from build123d import *

# Parameters (mm, degrees)
SKETCH1_R           = 275
BOSS_EXTRUDE1_DEPTH = 70
SKETCH2_R           = 275
SKETCH2_R_2         = 265
CUT_EXTRUDE1_DEPTH  = 10
SKETCH3_R           = 275
BOSS_EXTRUDE2_DEPTH = 50
SKETCH4_R           = 150
SKETCH4_R_2         = 100
BOSS_EXTRUDE3_DEPTH = 100
BOSS_EXTRUDE4_DEPTH = 100
FILLET3_R           = 20
BOSS_EXTRUDE5_DEPTH = 75
CUT_EXTRUDE4_DEPTH  = 150
CUT_EXTRUDE5_DEPTH  = 87.5


with BuildPart() as part:
    # Sketch1 → Boss-Extrude1 (new body)
    with BuildSketch(Plane.XY):
        Circle(SKETCH1_R)
    extrude(amount=BOSS_EXTRUDE1_DEPTH)

    # Sketch2 → Cut-Extrude1 (cut)
    with BuildSketch(Plane.XY.offset(70)):
        Circle(SKETCH2_R)
        Circle(SKETCH2_R_2, mode=Mode.SUBTRACT)
    extrude(amount=-CUT_EXTRUDE1_DEPTH, mode=Mode.SUBTRACT)

    # Sketch3 → Boss-Extrude2 (add)
    with BuildSketch(Plane.XY.offset(70)):
        Circle(SKETCH3_R)
    extrude(amount=BOSS_EXTRUDE2_DEPTH)



with BuildPart() as body_2:
    # Sketch4 → Boss-Extrude3 (new body, symmetric)
    with BuildSketch(Plane(origin=(0, 0, 0), x_dir=(0, 0, -1), z_dir=(1, 0, 0))):
        with Locations((-375, 0)):
            Circle(SKETCH4_R)
        with Locations((-375, 0)):
            Circle(SKETCH4_R_2, mode=Mode.SUBTRACT)
    extrude(amount=BOSS_EXTRUDE3_DEPTH, both=True)


with BuildPart() as part_1:
    add(part.part)

    add(body_2.part)  # Boss-Extrude4 merges body 2
    # Sketch6 → Boss-Extrude4 (add, symmetric)
    with BuildSketch(Plane(origin=(0, 0, 0), x_dir=(0, 0, -1), z_dir=(1, 0, 0))):
        with BuildLine():
            Line((-375, 150), (-120, 150))
            Line((-120, 150), (-120, -150))
            Line((-120, -150), (-375, -150))
            ThreePointArc((-375, -150), (-225, 0), (-375, 150))
        make_face()
    extrude(amount=BOSS_EXTRUDE4_DEPTH, both=True)

    # Fillet3
    fillet3_edges = [part_1.edges().sort_by_distance(p)[0] for p in [
        (-100, -150, 247.5),
        (-100, 150, 247.5),
        (100, -150, 247.5),
        (100, 150, 247.5),
        (-100, 0, 525),
        (100, 0, 525),
    ]]
    fillet(fillet3_edges, radius=FILLET3_R)

    # Sketch7 → Boss-Extrude5 (add)
    with BuildSketch(Plane.XY.offset(120)):
        with BuildLine():
            ThreePointArc((-266.057108103, 69.560155462), (-275, 0), (-266.057108103, -69.560155462))
            Line((-266.057108103, -69.560155462), (-100, -130))
            Line((-100, -130), (-100, 130))
            Line((-100, 130), (-266.057108103, 69.560155462))
        make_face()
        with BuildLine():
            Line((100, -130), (266.057108103, -69.560155462))
            ThreePointArc((266.057108103, -69.560155462), (272.755114277, -35.066331942), (275, 0))
            ThreePointArc((275, 0), (272.755114277, 35.066331942), (266.057108103, 69.560155462))
            Line((266.057108103, 69.560155462), (100, 130))
            Line((100, 130), (100, -130))
        make_face()
        with BuildLine():
            ThreePointArc((35.333334581, 272.72065464), (0, 275), (-35.333334581, 272.72065464))
            Line((-35.333334581, 272.72065464), (-80, 150))
            Line((-80, 150), (80, 150))
            Line((80, 150), (35.333334581, 272.72065464))
        make_face()
        with BuildLine():
            Line((80, -150), (-80, -150))
            Line((-80, -150), (-35.333334581, -272.72065464))
            ThreePointArc((-35.333334581, -272.72065464), (0, -275), (35.333334581, -272.72065464))
            Line((35.333334581, -272.72065464), (80, -150))
        make_face()
    extrude(amount=BOSS_EXTRUDE5_DEPTH)

    # Sketch8 → Cut-Extrude4 (cut, symmetric)
    with BuildSketch(Plane(origin=(0, 0, 0), x_dir=(1, 0, 0), z_dir=(0, 1, 0))):
        Polygon((-300, -120), (-100, -195), (-300, -195), align=None)
        Polygon((300, -120), (100, -195), (300, -195), align=None)
    extrude(amount=CUT_EXTRUDE4_DEPTH, both=True, mode=Mode.SUBTRACT)

    # Sketch9 → Cut-Extrude5 (cut, symmetric)
    with BuildSketch(Plane(origin=(0, 0, 0), x_dir=(0, 0, -1), z_dir=(1, 0, 0))):
        Polygon((-195, 150), (-195, 290), (-120, 290), align=None)
        Polygon((-120, -290), (-195, -150), (-195, -290), align=None)
    extrude(amount=CUT_EXTRUDE5_DEPTH, both=True, mode=Mode.SUBTRACT)


solid = part_1.part
Verification items for the finished model (mm, model axes). A direction names the side the tool comes from. Give positions to 0.01 mm unless a question says otherwise; leave off trailing zeros. Write each loop counter-clockwise with the first axis right and the second up, starting at its lowest first coordinate (ties: lowest second). Pieces come first, ordered by that corner, then holes. Notation, with made-up numbers: (-8, 22.25) - (14, 22.25) arc R32 cw to (14, 56.25) - close; hole circle Ø2 at (83.25, 23.25). An arc over 180 degrees is marked (long way). Answer as CSV lines item,"result". Start each with the question number.
1. Sectioned sample at C-C (y = 161.5). Record the boundary of the cut face in (x, z), then the cut area to 3 significant figures.
2. Sectioned sample at A-A (x = 0). Record the boundary of the cut face in (y, z), then the cut area to 3 significant figures.
3. Depth check by flat-ended pin: pin 1 (1 mm diameter, centred on y = 189.5, z = 64, fed in from +X); pin 2 (1 mm diameter, centred on x = 26.5, z = 380.5, fed in from -Y); pin 3 (1 mm diameter, centred on x = -28.5, y = -108, fed in from +Z). Enter the tip coordinate at first touch or a pass-through.
4. Draft check along Z on faces 5 (the face through (-1.4, -60.848, 454.357)), 6 (the face through (149, -170, 120)), 7 (the face through (1, -150, 284)). Enter one of: pulls with the +Z half, pulls with the -Z half, needs draft (parallel to the pull), parting line crosses it, or undercut.
5. Thickness scan on line 1 (Y direction, x = -7, z = 375); line 2 (Z direction, x = -162.5, y = -195); line 3 (X direction, y = 91.5, z = 301). Record the ranges inside material, lowest first.
6. Sectioned sample at B-B (z = 205.5). Record the boundary of the cut face in (x, y).
7. Sectioned sample at D-D (x = -189.5). Record the boundary of the cut face in (y, z).
8. Set-up check for faces 1 (the face through (142.46, 223.45, 65.07)), 2 (the face through (-62.32, 198.58, 148.64)), 3 (the face through (-100, 31, 279)), 4 (the face through (-165.74, -106.073, 148.642)): record each of +Z, -Z, +X, -X, +Y, -Y from which the full face is reachable in a straight line by a thin tool's end or side.
Derived:
1,outline,"(-222.58, 0) - (222.58, 0) - (222.58, 60) - (210.1, 60) - (210.1, 70) - (222.58, 70) - (222.58, 120) - (75.81, 120) - (75.81, 188.84) - (-75.81, 188.84) - (-75.81, 120) - (-222.58, 120) - (-222.58, 70) - (-210.1, 70) - (-210.1, 60) - (-222.58, 60) - close"
1,area,"63,600 mm²"
2,outline,"(-275, 0) - (275, 0) - (275, 60) - (265, 60) - (265, 70) - (275, 70) - (275, 128.04) - (150, 195) - (150, 375) arc R150 ccw to (-150, 375) - (-150, 195) - (-275, 128.04) - (-275, 70) - (-265, 70) - (-265, 60) - (-275, 60) - close; hole circle Ø200 at (0, 375)"
2,area,"157,000 mm²"
3,pin 1,"x = 185.75"
3,pin 2,"y = -149.92"
3,pin 3,"z = 479.61"
4,face 5,"undercut"
4,face 6,"pulls with the +Z half"
4,face 7,"needs draft"
5,line 1,"-150 to -100, 100 to 150"
5,line 2,"0 to 120"
5,line 3,"-100 to 100"
6,outline,"(-100, -130) arc R20 ccw to (-80, -150) - (80, -150) arc R20 ccw to (100, -130) - (100, 130) arc R20 ccw to (80, 150) - (-80, 150) arc R20 ccw to (-100, 130) - close"
7,outline,"(-199.29, 0) - (199.29, 0) - (199.29, 60) - (185.24, 60) - (185.24, 70) - (199.29, 70) - (199.29, 120) - (97.42, 120) - (97.42, 161.44) - (-97.42, 161.44) - (-97.42, 120) - (-199.29, 120) - (-199.29, 70) - (-185.24, 70) - (-185.24, 60) - (-199.29, 60) - close"
8,face 1,"none"
8,face 2,"+Z, -X, +Y"
8,face 3,"+Z, -X, +Y, -Y"
8,face 4,"+Z, -X, -Y"
